```python
from build123d import *

# Parameters (mm, degrees)
F1_R     = 44.522092
F2_DEPTH = 34.475029
F3_SIZE  = 6.35
F4_SIZE  = 5.08


with BuildPart() as f2:
    # F1 (on face) → F2 (new body)
    with BuildSketch(Plane.XY):
        Polygon((-33.91923, -58.74983), (33.91923, -58.74983), (67.83846, 0), (33.91923, 58.74983), (-33.91923, 58.74983), (-67.83846, 0), align=None)
        Circle(F1_R, mode=Mode.SUBTRACT)
    extrude(amount=F2_DEPTH)

    # F3
    f3_edges = [f2.edges().sort_by_distance(p)[0] for p in [
        (0, 58.74983, 34.475029),
        (-50.878845, -29.374915, 34.475029),
        (50.878845, 29.374915, 34.475029),
        (0, -58.74983, 34.475029),
        (50.878845, -29.374915, 34.475029),
        (-50.878845, 29.374915, 34.475029),
    ]]
    chamfer(f3_edges, length=F3_SIZE)

    # F4
    f4_edges = [f2.edges().sort_by_distance(p)[0] for p in [
        (50.878845, -29.374915, 0),
        (50.878845, 29.374915, 0),
        (0, 58.74983, 0),
        (-50.878845, 29.374915, 0),
        (-50.878845, -29.374915, 0),
        (0, -58.74983, 0),
        (-44.522092, 0, 0),
    ]]
    chamfer(f4_edges, length=F4_SIZE)


solid = f2.part
```
Part model, mm, in its own coordinate system. Round coordinates to 2 decimals unless told otherwise and drop trailing zeros. Order: outer loops, then holes, each group sorted by start corner. A loop starts at its lowest first (then second) coordinate and runs counter-clockwise, first axis right, second up. Notation, with made-up numbers: M 21.5,12.5 L 50.5,12.5 A19 cw 50.5,26.5 Z; hole C -1.75,15 d6. An arc over 180 degrees is marked long. Put each result on its own line as item: value. Start each with the question number.
1. Slice it at C-C on x = 58.5. List the corners of the cut face in (y, z).
2. Drill centre lines: probe 1 along Y at (x, z) = (0, 19); probe 2 along Y at (x, z) = (-35, 19); probe 3 along X at (y, z) = (-18, 26.5). Where is each one in solid material? Low to high. Write a range as [from, to].
3. Two-plate mould, pull along Y, no slides. Class faces 1 (the face through (0.475, 55.53, 31.344)), 2 (the face through (42.466, 13.373, 19.572)), 3 (the face through (50.64, -29.79, 16.44)), 4 (the face through (42.701, 13.447, 4.833)): +Y half, -Y half, draft (parallel to the pull), parting line (faces both ways), or undercut.
4. Drop flat-ended pins along their axis: pin 1 (3 mm diameter, centred on y = -35, z = 8, fed in from -X); pin 2 (5 mm diameter, centred on y = 42.5, z = 19, fed in from -X); pin 3 (6 mm diameter, centred on x = 3, y = 41.5, fed in from -Z). Give the stop position or say it passes through.
5. Slice it at A-A on x = 0. List the corners of the cut face in (y, z).
6. Slice it at B-B on z = 9. List the corners of the cut face in (x, y).
Findings:
1. outline: M -16.17,5.08 L -6.01,0 L 6.01,0 L 16.17,5.08 L 16.17,28.13 L 3.47,34.48 L -3.47,34.48 L -16.17,28.13 Z
2. probe 1: [-58.75, -44.52], [44.52, 58.75]
2. probe 2: [-56.88, -27.52], [27.52, 56.88]
2. probe 3: [-57.45, -40.72], [40.72, 57.45]
3. face 1: +Y half
3. face 2: undercut
3. face 3: -Y half
3. face 4: undercut
4. pin 1: x = -48.5
4. pin 2: x = -44.74
4. pin 3: z = 4.99
5. outline: M -58.75,5.08 L -53.67,0 L -49.6,0 L -44.52,5.08 L -44.52,34.48 L -52.4,34.48 L -58.75,28.13 Z; M 44.52,5.08 L 49.6,0 L 53.67,0 L 58.75,5.08 L 58.75,28.13 L 52.4,34.48 L 44.52,34.48 Z
6. outline: M -67.84,0 L -33.92,-58.75 L 33.92,-58.75 L 67.84,0 L 33.92,58.75 L -33.92,58.75 Z; hole C 0,0 d89.04
